For this review, take the finished solid that the model builds, in its own axes (mm). A direction names the side the tool comes from. Coordinates: 2 decimals unless noted, no trailing zeros. Order: outer loops, then holes, each group sorted by start corner. A loop starts at its lowest first (then second) coordinate and runs counter-clockwise, first axis right, second up. Notation, with made-up numbers: (-35.75, 83.5) -> (-20.75, 83.5) arc R24 ccw to (-20.75, 116.5) -> close; hole circle Ø5 at (43, 86). An arc over 180 degrees is marked (long way). Answer as a JSON object with one key per item and string values. Group by question number.
1) Machinability: for faces 4 (the conical face through (3.34, 8, 12.55)), 5 (the cylindrical face through (-5.341, -26.054, 7.084)), 6 (the cylindrical face through (1.44, -12.19, 0.54)), which of the approach directions +Z, -Z, +X, -X, +Y, -Y give a long, thin tool a straight path to every point of the face, cutting with its end or side? Answer none if there is none.
2) For pin 1 (5 mm diameter, centred on x = 4, y = 4.5, fed in from +Z); pin 2 (12 mm diameter, centred on y = -20.5, z = 17, fed in from +X); pin 3 (1.4 mm diameter, centred on x = -5.5, z = 24.5, fed in from +Y), all flat-tipped, find the tip position at first contact; note any pin that passes through.
3) Draft analysis for pull direction Y (two halves, no side actions). For faces 1 (the flat face through (-5, -23, 0)), 2 (the flat face through (-4.7, -13, 13)), 3 (the conical face through (-3.32, -11.78, -9.03)), state which applies: +Y half, -Y half, draft (parallel to the pull), parting line (faces both ways), or undercut.
4) Add section A-A, the plane y = 20.5. Write out the cut boundary in (x, z), then the cut area to 3 significant figures.
5) Wall thickness on L1, parallel to Z at x = 2, y = 0; L2, parallel to X at y = -10, z = 4.5; L3, parallel to X at y = 24.5, z = 11.5: over which ranges is each line inside the solid? List them lowest first.
6) Add section D-D, the plane z = -7.5. Count the separate pieces of the cut face and the enclosed holes in it, then the cut area to 3 significant figures.
7) Add section B-B, the plane z = 21.5. Write out the cut boundary in (x, y).
8) Add section C-C, the plane x = 2. Write out the cut boundary in (y, z), then the cut area to 3 significant figures.
from build123d import *

# Parameters (mm, degrees)
SKETCH001_R        = 28
SKETCH001_R_2      = 17.7
PAD_DEPTH          = 1.3
POCKET_DEPTH       = 159.714257
POLARPATTERN_COUNT = 4


with BuildPart() as body001:
    # Sketch001 → Pad (new body)
    with BuildSketch(Plane.YZ):
        Circle(SKETCH001_R)
        Circle(SKETCH001_R_2, mode=Mode.SUBTRACT)
    extrude(amount=PAD_DEPTH)

    # Sketch002 (on Face4 of Pad) → Pocket (cut, through all)
    with BuildSketch(Plane.YZ.offset(1.3)):
        with BuildLine():
            ThreePointArc((-23.382686, 13.5), (-26.079997, 6.988114), (-27, 0))
            Line((-27, 0), (-18, 0))
            ThreePointArc((-15.588457, 9), (-17.386665, 4.658743), (-18, 0))
            Line((-23.382686, 13.5), (-15.588457, 9))
        make_face()
    pocket = extrude(amount=-POCKET_DEPTH, mode=Mode.SUBTRACT)

    # PolarPattern: Pocket ×4 about axis
    polarpattern_axis = Axis((0, 0, 0), (1, 0, 0))
    for i in range(1, POLARPATTERN_COUNT):
        add(pocket.rotate(polarpattern_axis, i * 360 / POLARPATTERN_COUNT), mode=Mode.SUBTRACT)


with BuildPart() as body001_1:
    # Body001 placement: moved
    add(body001.part.moved(Location((-6, 0, 0))))


with BuildPart() as fusion:
    # Sketch → Revolution (revolve)
    with BuildSketch(Plane.XY):
        Polygon((-6, 12.2), (-6, 17.7), (-4.717735, 17.7), (-3.25, 14.7), (3.25, 14.7), (4.717735, 17.7), (6, 17.7), (6, 12.2), (-3, 12.2), (-3, 10.7), (-6, 10.7), align=None)
    revolve(axis=Axis((0, 0, 0), (1, 0, 0)))

    # Fusion: union Body001
    add(body001_1.part)


solid = fusion.part
Output values:
{
 "1": {"face 4": "none", "face 5": "+X, -X", "face 6": "+X"},
 "2": {"pin 1": "stops at z = 17.57", "pin 2": "stops at x = -4.7", "pin 3": "stops at y = 14.75"},
 "3": {"face 1": "undercut", "face 2": "draft", "face 3": "parting line"},
 "4": {"outline": "(-6, -19.07) -> (-4.7, -19.07) -> (-4.7, -11.84) -> (-6, -11.84) -> close; (-6, 0) -> (-4.7, 0) -> (-4.7, 19.07) -> (-6, 19.07) -> close", "area": "34.2 mm²"},
 "5": {"L1": "z = -14.7 to -12.2, 12.2 to 14.7", "L2": "x = -6 to -3", "L3": "x = -6 to -4.7"},
 "6": {"separate pieces": "3", "enclosed holes": "0", "area": "128 mm²"},
 "7": {"outline": "(-6, -17.94) -> (-4.7, -17.94) -> (-4.7, 0) -> (-6, 0) -> close; (-6, 12.41) -> (-4.7, 12.41) -> (-4.7, 17.94) -> (-6, 17.94) -> close"},
 "8": {"outline": "circle Ø29.4 at (0, 0); hole circle Ø24.4 at (0, 0)", "area": "211 mm²"}
}
